```python
from build123d import *

# Parameters (mm, degrees)
SKETCH1_W           = 60
SKETCH1_H           = 40
SKETCH1_R           = 2.5
BOSS_EXTRUDE3_DEPTH = 30
SKETCH4_W           = 50
SKETCH4_H           = 30
CUT_EXTRUDE1_DEPTH  = 20
SKETCH5_R           = 2.5
CUT_EXTRUDE4_DEPTH  = 49


with BuildPart() as part:
    # Sketch1 → Boss-Extrude3 (new body)
    with BuildSketch(Plane.XY):
        Rectangle(SKETCH1_W, SKETCH1_H)
        with Locations((-17.5, 7.5)):
            Circle(SKETCH1_R, mode=Mode.SUBTRACT)
        with Locations((17.5, 7.5)):
            Circle(SKETCH1_R, mode=Mode.SUBTRACT)
        with Locations((-17.5, -7.5)):
            Circle(SKETCH1_R, mode=Mode.SUBTRACT)
        with Locations((17.5, -7.5)):
            Circle(SKETCH1_R, mode=Mode.SUBTRACT)
    extrude(amount=BOSS_EXTRUDE3_DEPTH)

    # Sketch4 → Cut-Extrude1 (cut)
    with BuildSketch(Plane.XY.offset(30)):
        Rectangle(SKETCH4_W, SKETCH4_H)
    extrude(amount=-CUT_EXTRUDE1_DEPTH, mode=Mode.SUBTRACT)

    # Sketch5 → Cut-Extrude4 (cut)
    with BuildSketch(Plane(origin=(0, 20, 0), x_dir=(1, 0, 0), z_dir=(0, 1, 0))):
        with Locations((-17.5, -10)):
            Circle(SKETCH5_R)
        with Locations((17.5, -10)):
            Circle(SKETCH5_R)
        with Locations((17.5, -25)):
            Circle(SKETCH5_R)
        with Locations((-17.5, -25)):
            Circle(SKETCH5_R)
    extrude(amount=-CUT_EXTRUDE4_DEPTH, mode=Mode.SUBTRACT)


solid = part.part
```
Check sheet for the modelled part. Datum: model origin and axes. Units: mm. A direction names the side the tool comes from. Round coordinates to 2 decimals unless told otherwise and drop trailing zeros. Order: outer loops, then holes, each group sorted by start corner. A loop starts at its lowest first (then second) coordinate and runs counter-clockwise, first axis right, second up. Notation, with made-up numbers: (16, 76.25) - (29, 76.25) arc R6 cw to (29, 87.25) - close; hole circle Ø5 at (37.5, -14). An arc over 180 degrees is marked (long way). Write item = value, one per line.
Q1. Section check B-B (x = -17.5). Record the boundary of the cut face in (y, z).
Computed:
outline = (-20, 0) - (-10, 0) - (-10, 7.5) - (-20, 7.5) - close; (-20, 12.5) - (-15, 12.5) - (-15, 22.5) - (-20, 22.5) - close; (-20, 27.5) - (-15, 27.5) - (-15, 30) - (-20, 30) - close; (-5, 0) - (5, 0) - (5, 7.5) - (-5, 7.5) - close; (10, 0) - (20, 0) - (20, 7.5) - (10, 7.5) - close; (15, 12.5) - (20, 12.5) - (20, 22.5) - (15, 22.5) - close; (15, 27.5) - (20, 27.5) - (20, 30) - (15, 30) - close
Q2. Section check A-A (z = 4.25). Record the boundary of the cut face in (x, y), and give its area (3 significant figures).
Computed:
outline = (-30, -20) - (30, -20) - (30, 20) - (-30, 20) - close; hole circle Ø5 at (-17.5, -7.5); hole circle Ø5 at (-17.5, 7.5); hole circle Ø5 at (17.5, -7.5); hole circle Ø5 at (17.5, 7.5)
area = 2,320 mm^2
Q3. Draft check along Y on faces 3 (the face through (0, 15, 20)), 4 (the face through (0, 0, 0)), 5 (the face through (0, -20, 15)). Enter one of: pulls with the +Y half, pulls with the -Y half, needs draft (parallel to the pull), parting line crosses it, or undercut.
Computed:
face_3 = undercut
face_4 = needs draft
face_5 = pulls with the -Y half
Q4. Section check C-C (z = 25). Record the boundary of the cut face in (x, y), and give its area (3 significant figures).
Computed:
outline = (-30, -20) - (-20, -20) - (-20, -15) - (-25, -15) - (-25, 15) - (-20, 15) - (-20, 20) - (-30, 20) - close; (-15, -20) - (15, -20) - (15, -15) - (-15, -15) - close; (-15, 15) - (15, 15) - (15, 20) - (-15, 20) - close; (20, -20) - (30, -20) - (30, 20) - (20, 20) - (20, 15) - (25, 15) - (25, -15) - (20, -15) - close
area = 800 mm^2
Q5. Tool access check on faces 1 (the face through (-17.83, -15.05, 7.52)), 2 (the face through (0, -15, 20)). Record the directions out of +Z, -Z, +X, -X, +Y, -Y that give a thin tool (end or side, any length) a straight path to the whole face; none if there is none.
Computed:
face_1 = +Y, -Y
face_2 = +Z
Q6. Section check D-D (y = 3). Record the boundary of the cut face in (x, z), and give its area (3 significant figures).
Computed:
outline = (-30, 0) - (30, 0) - (30, 30) - (25, 30) - (25, 10) - (20, 10) arc R2.5 cw to (15, 10) - (-15, 10) arc R2.5 cw to (-20, 10) - (-25, 10) - (-25, 30) - (-30, 30) - close
area = 780 mm^2
Q7. Thickness scan on line 1 along Z through (x, y) = (-17.5, -17.65); line 2 along X through (y, z) = (-17.3, 25); line 3 along Y through (x, z) = (-17.5, 4.5). Record the ranges inside material, lowest first.
Computed:
line_1 = 0 to 7.5, 12.5 to 22.5, 27.5 to 30
line_2 = -30 to -20, -15 to 15, 20 to 30
line_3 = -20 to -10, -5 to 5, 10 to 20
Q8. Go/stop test with a flat-tipped pin: pin 1 (4 mm diameter, centred on x = 16.5, y = -7, fed in from +Z). Record where the tip stops, or that it passes through.
Computed:
pin_1 = 10
